Read the model definition and answer for the solid it produces. Units are mm, in the model's axes. Face numbers are marked on the shaded views. A direction names the side the tool comes from. Coordinates: 2 decimals unless noted, no trailing zeros. Write each loop counter-clockwise with the first axis right and the second up, starting at its lowest first coordinate (ties: lowest second). Pieces come first, ordered by that corner, then holes.
(1) Given pin 1 (8 mm diameter, centred on x = 43.5, z = 11, fed in from +Y); pin 2 (1 mm diameter, centred on x = 6.5, z = 3, fed in from -Y); pin 3 (5 mm diameter, centred on x = 24, z = 20.5, fed in from -Y); pin 4 (3 mm diameter, centred on y = -8, z = 15, fed in from +X), each flat-ended and moving along its own axis, determine where each tip first touches the part or whether it passes through.
(2) The mould has two halves that part along Z. Classify the marked faces 4, 5, 6 and 7: +Z half, -Z half, draft (parallel to the pull), parting line (faces both ways), or undercut.
(3) Which of the six approach directions +Z, -Z, +X, -X, +Y, -Y give full straight-line access (tool end or side, diameter ignored) to the marked faces 1, 2 and 3?
(4) Section D-D on z = 17 is taken. Write down the section's boundary in (x, y), then the cut area to 3 significant figures.
(5) Section C-C on x = 29 is taken. Write down the section's boundary in (y, z).
(6) Find the intervals of material crossed by probe 1 along Y at (x, z) = (13, 0); probe 2 along Y at (x, z) = (33, 4.5); probe 3 along Z at (x, y) = (13, 6.5), in increasing order.
(7) Section B-B on z = 0 is taken. Write down the section's boundary in (x, y).
(8) Section A-A on y = 0 is taken. Write down the section's boundary in (x, z).
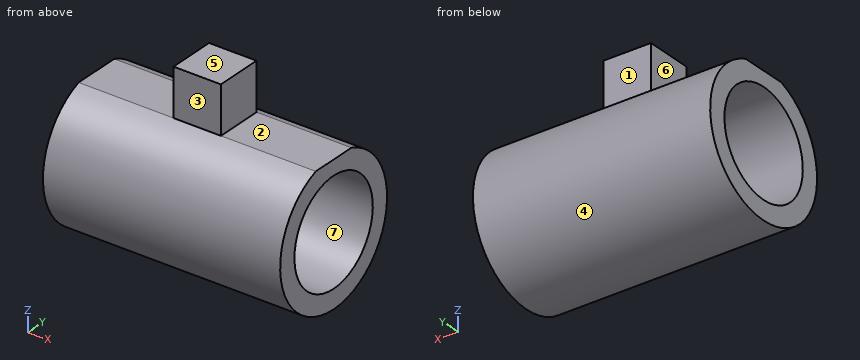
from build123d import *

# Parameters (mm, degrees)
SKETCH_1_R          = 15
SKETCH_1_R_2        = 11
EXTRUDE_1_DEPTH     = 50
SKETCH_2_W          = 10
SKETCH_2_H          = 10
EXTRUDE_2_DEPTH     = 50
SKETCH_3_W          = 20
SKETCH_3_H          = 10
CUT_EXTRUDE_1_DEPTH = 50


with BuildPart() as part:
    # 草图1 → 凸台-拉伸1 (new body)
    with BuildSketch(Plane(origin=(0, 0, 0), x_dir=(0, 0, -1), z_dir=(1, 0, 0))):
        Circle(SKETCH_1_R)
        Circle(SKETCH_1_R_2, mode=Mode.SUBTRACT)
    extrude(amount=EXTRUDE_1_DEPTH)

    # 草图2 → 凸台-拉伸2 (add)
    with BuildSketch(Plane.ZY):
        with Locations((19.142135624, 0)):
            Rectangle(SKETCH_2_W, SKETCH_2_H)
    extrude(amount=-EXTRUDE_2_DEPTH)

    # 草图3 → 切除-拉伸1 (cut)
    with BuildSketch(Plane(origin=(0, -5, 0), x_dir=(-1, 0, 0), z_dir=(0, -1, 0))):
        with Locations((-10, -19.142135624)):
            Rectangle(SKETCH_3_W, SKETCH_3_H)
        with Locations((-40, -19.142135624)):
            Rectangle(SKETCH_3_W, SKETCH_3_H)
    extrude(amount=-CUT_EXTRUDE_1_DEPTH, mode=Mode.SUBTRACT)


solid = part.part
Response:
1. pin 1: stops at y = 13.27
1. pin 2: stops at y = -14.79
1. pin 3: stops at y = -5
1. pin 4: passes through
2. face 4: parting line
2. face 5: +Z half
2. face 6: draft
2. face 7: undercut
3. face 1: +Z, +X, -X, +Y
3. face 2: +Z, +X, +Y, -Y
3. face 3: +Z, +X, -X, -Y
4. outline: (20, -5) - (30, -5) - (30, 5) - (20, 5) - close
4. area: 100 mm2
5. outline: (-5, 14.14) arc R15 ccw (long way) to (5, 14.14) - (5, 24.14) - (-5, 24.14) - close; hole circle Ø22 at (0, 0)
6. probe 1: y = -15 to -11, 11 to 15
6. probe 2: y = -14.31 to -10.04, 10.04 to 14.31
6. probe 3: z = -13.52 to -8.87, 8.87 to 13.52
7. outline: (0, -15) - (50, -15) - (50, -11) - (0, -11) - close; (0, 11) - (50, 11) - (50, 15) - (0, 15) - close
8. outline: (0, -15) - (50, -15) - (50, -11) - (0, -11) - close; (0, 11) - (50, 11) - (50, 14.14) - (30, 14.14) - (30, 24.14) - (20, 24.14) - (20, 14.14) - (0, 14.14) - close
